from build123d import *

# Parameters (mm, degrees)
SKETCH_1_R      = 4
SKETCH_1_R_2    = 2
SKETCH_1_R_3    = 1.5
SKETCH_1_W      = 10
SKETCH_1_H      = 5
SKETCH_1_H_2    = 32.3
EXTRUDE_1_DEPTH = 5


with BuildPart() as part:
    # 草图1 → 凸台-拉伸1 (new body)
    with BuildSketch(Plane(origin=(0, 0, 0), x_dir=(1, 0, 0), z_dir=(0, 1, 0))):
        with BuildLine():
            Line((10, 5), (10, 10))
            Line((10, 10), (30, 10))
            Line((30, 10), (30, 5))
            ThreePointArc((30, 5), (31.464466094, 1.464466094), (35, 0))
            Line((35, 0), (40, 0))
            Line((40, 0), (40, 115))
            Line((40, 115), (45, 115))
            Line((45, 115), (45, 125))
            Line((45, 125), (40, 125))
            Line((40, 125), (40, 135))
            Line((40, 135), (45, 135))
            Line((45, 135), (45, 145))
            Line((45, 145), (40, 145))
            Line((40, 145), (40, 150))
            Line((40, 150), (35, 150))
            Line((35, 150), (35, 145))
            Line((35, 145), (25, 145))
            Line((25, 145), (25, 150))
            Line((25, 150), (20, 150))
            ThreePointArc((20, 150), (5.857864376, 144.142135624), (0, 130))
            Line((0, 130), (0, 0))
            Line((0, 0), (5, 0))
            ThreePointArc((5, 0), (8.535533906, 1.464466094), (10, 5))
        make_face()
        with Locations(Location((20, 138, 0), (0, 0, 270))):
            Circle(SKETCH_1_R, mode=Mode.SUBTRACT)
        with Locations(Location((20, 106, 0), (0, 0, 270))):
            Circle(SKETCH_1_R, mode=Mode.SUBTRACT)
        with Locations(Location((20, 124, 0), (0, 0, 270))):
            Circle(SKETCH_1_R_2, mode=Mode.SUBTRACT)
        with Locations(Location((20, 88, 0), (0, 0, 270))):
            Circle(SKETCH_1_R_2, mode=Mode.SUBTRACT)
        with Locations(Location((8.5, 42.3, 0), (0, 0, 270))):
            Circle(SKETCH_1_R_3, mode=Mode.SUBTRACT)
        with Locations(Location((31.5, 42.3, 0), (0, 0, 270))):
            Circle(SKETCH_1_R_3, mode=Mode.SUBTRACT)
        with Locations(Location((8.5, 20, 0), (0, 0, 270))):
            Circle(SKETCH_1_R_3, mode=Mode.SUBTRACT)
        with Locations(Location((31.5, 20, 0), (0, 0, 270))):
            Circle(SKETCH_1_R_3, mode=Mode.SUBTRACT)
        with Locations((10, 78.5)):
            Rectangle(SKETCH_1_W, SKETCH_1_H, mode=Mode.SUBTRACT)
        with Locations((30, 78.5)):
            Rectangle(SKETCH_1_W, SKETCH_1_H, mode=Mode.SUBTRACT)
        with Locations((20, 31.15)):
            Rectangle(SKETCH_1_W, SKETCH_1_H_2, mode=Mode.SUBTRACT)
    extrude(amount=EXTRUDE_1_DEPTH)


solid = part.part
The model under review builds one solid part; all positions refer to its coordinate system, in mm. A direction names the side the tool comes from. Round coordinates to 2 decimals unless told otherwise and drop trailing zeros. Order: outer loops, then holes, each group sorted by start corner. A loop starts at its lowest first (then second) coordinate and runs counter-clockwise, first axis right, second up. Notation, with made-up numbers: (27, -9) -> (43, -9) arc R20 cw to (43, 22) -> close; hole circle Ø1 at (18.5, -17.75). An arc over 180 degrees is marked (long way). Use CSV: the item, a comma, the result in double quotes. Start each with the question number.
(1) Wall thickness on probe 1 along X at (y, z) = (1.3, -20); probe 2 along X at (y, z) = (1.45, -106); probe 3 along X at (y, z) = (3.2, -124): over which ranges is each line inside the solid? List them lowest first. Write a range as from..to.
(2) Mouldability with a two-part tool opening along X and no side actions: class faces 1 (the face through (20, 2, -126)), 2 (the face through (22, 5, -93)), 3 (the face through (0, 2, -66)) as pulls with the +X half, pulls with the -X half, needs draft (parallel to the pull), parting line crosses it, or undercut.
(3) Consider section B-B on z = -106. Write out the cut boundary in (x, y).
(4) Consider section D-D on x = 8.5. Write out the cut boundary in (y, z).
(5) Tool access review of faces 4 (the face through (42, 2, -135)), 5 (the face through (30, 2, -145)), 6 (the face through (5, 2, -78)), 7 (the face through (30, 2, -8)): name each direction out of +Z, -Z, +X, -X, +Y, -Y from which nothing blocks a thin tool from reaching the whole face with its end or side.
(6) Insertion check: pin 1 (4 mm diameter, centred on x = 31.5, z = -42.3, fed in from +Y); pin 2 (2.5 mm diameter, centred on x = 30, y = 3.5, fed in from -Z); pin 3 (2 mm diameter, centred on x = 20, y = 2.5, fed in from +Z); pin 4 (1.5 mm diameter, centred on y = 2.5, z = -148, fed in from -X). Each pin has a flat end and moves straight along its axis. Give the tip position at first contact, or say it passes through.
(7) Consider section C-C on z = -20. Write out the cut boundary in (x, y).
(8) Consider section A-A on x = 28. Write out the cut boundary in (y, z), and give its area (3 significant figures).
Responses:
1,probe 1,"0..7, 10..15, 25..30, 33..40"
1,probe 2,"0..16, 24..40"
1,probe 3,"0..18, 22..45"
2,face 1,"undercut"
2,face 2,"needs draft"
2,face 3,"pulls with the -X half"
3,outline,"(0, 0) -> (16, 0) -> (16, 5) -> (0, 5) -> close; (24, 0) -> (40, 0) -> (40, 5) -> (24, 5) -> close"
4,outline,"(0, -146.36) -> (5, -146.36) -> (5, -81) -> (0, -81) -> close; (0, -76) -> (5, -76) -> (5, -43.8) -> (0, -43.8) -> close; (0, -40.8) -> (5, -40.8) -> (5, -21.5) -> (0, -21.5) -> close; (0, -18.5) -> (5, -18.5) -> (5, -1.43) -> (0, -1.43) -> close"
5,face 4,"+X, +Y, -Y"
5,face 5,"-Z, +Y, -Y"
5,face 6,"+Y, -Y"
5,face 7,"+Z, +Y, -Y"
6,pin 1,"y = 5"
6,pin 2,"z = -145"
6,pin 3,"z = -10"
6,pin 4,"x = 9.88"
7,outline,"(0, 0) -> (7, 0) -> (7, 5) -> (0, 5) -> close; (10, 0) -> (15, 0) -> (15, 5) -> (10, 5) -> close; (25, 0) -> (30, 0) -> (30, 5) -> (25, 5) -> close; (33, 0) -> (40, 0) -> (40, 5) -> (33, 5) -> close"
8,outline,"(0, -145) -> (5, -145) -> (5, -81) -> (0, -81) -> close; (0, -76) -> (5, -76) -> (5, -10) -> (0, -10) -> close"
8,area,"650 mm²"
